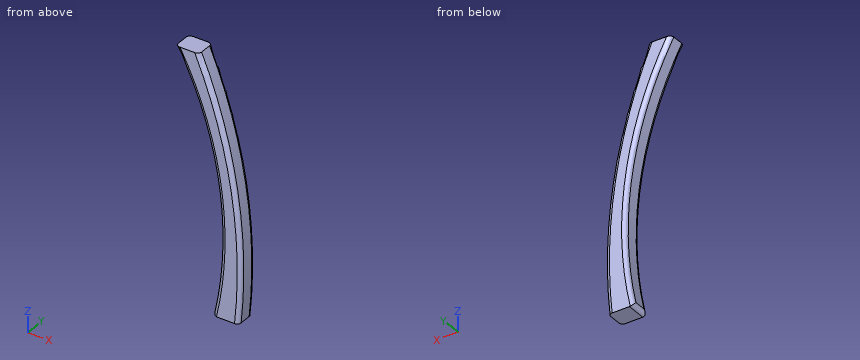
```python
from build123d import *

# Parameters (mm, degrees)
F1_DEPTH = 25.4
F2_R     = 5.08


with BuildPart() as f1:
    # F0 (on Front) → F1 (new body)
    with BuildSketch(Plane.XZ):
        with BuildLine():
            Line((-46.963625, -95.087554), (-13.032385, -95.087554))
            ThreePointArc((-13.032385, -95.087554), (-17.386338, 72.400967), (-64.540181, 233.173716))
            Line((-64.540181, 233.173716), (-95.020181, 233.173716))
            ThreePointArc((-95.020181, 233.173716), (-40.436227, 73.516349), (-46.963625, -95.087554))
        make_face()
    extrude(amount=F1_DEPTH)

    # F2
    f2_edges = [f1.edges().sort_by_distance(p)[0] for p in [
        (-40.436227, 0, 73.516349),
        (-46.963625, -12.7, -95.087554),
        (-17.386338, -25.4, 72.400967),
        (-40.436227, -25.4, 73.516349),
        (-17.386338, 0, 72.400967),
    ]]
    fillet(f2_edges, radius=F2_R)


solid = f1.part
```
The model under review builds one solid part; all positions refer to its coordinate system, in mm. Give positions to 0.01 mm unless a question says otherwise; leave off trailing zeros. Write each loop counter-clockwise with the first axis right and the second up, starting at its lowest first coordinate (ties: lowest second). Pieces come first, ordered by that corner, then holes. Notation, with made-up numbers: M 19,-33 L 56,-33 A5 cw 56,-29 Z; hole C 84.5,85.5 d2. An arc over 180 degrees is marked long. Write each question's results on one line, items separated by ' | '. Start each with the question number.
1. For probe 1 along X at (y, z) = (-15, 108.5); probe 2 along X at (y, z) = (-4, 64); probe 3 along Z at (x, y) = (-86, -4.5), list the stretches that pass through material, from the lowest coordinate up. Write a range as [from, to].
2. We need section A-A (y = -12). Write out the cut boundary in (x, z).
3. Insertion check: pin 1 Ø4 at (y, z) = (-15.5, 138) entering from +X; pin 2 Ø5 at (y, z) = (-9.5, 6.5) entering from +X; pin 3 Ø12 at (y, z) = (-7, 161.5) entering from +X. Each pin has a flat end and moves straight along its axis. Give the tip position at first contact, or say it passes through.
Results found:
1) probe 1: x = [-46.95, -24.1] | probe 2: x = [-39.03, -16.24] | probe 3: z = [216.45, 233.17]
2) outline: M -95.02,233.17 A460.96 cw -45.62,-88.95 A5.08 ccw -40.65,-95.09 L -13.03,-95.09 A647.95 ccw -64.54,233.17 Z
3) pin 1: stops at x = -30.66 | pin 2: stops at x = -10.35 | pin 3: stops at x = -36.09
